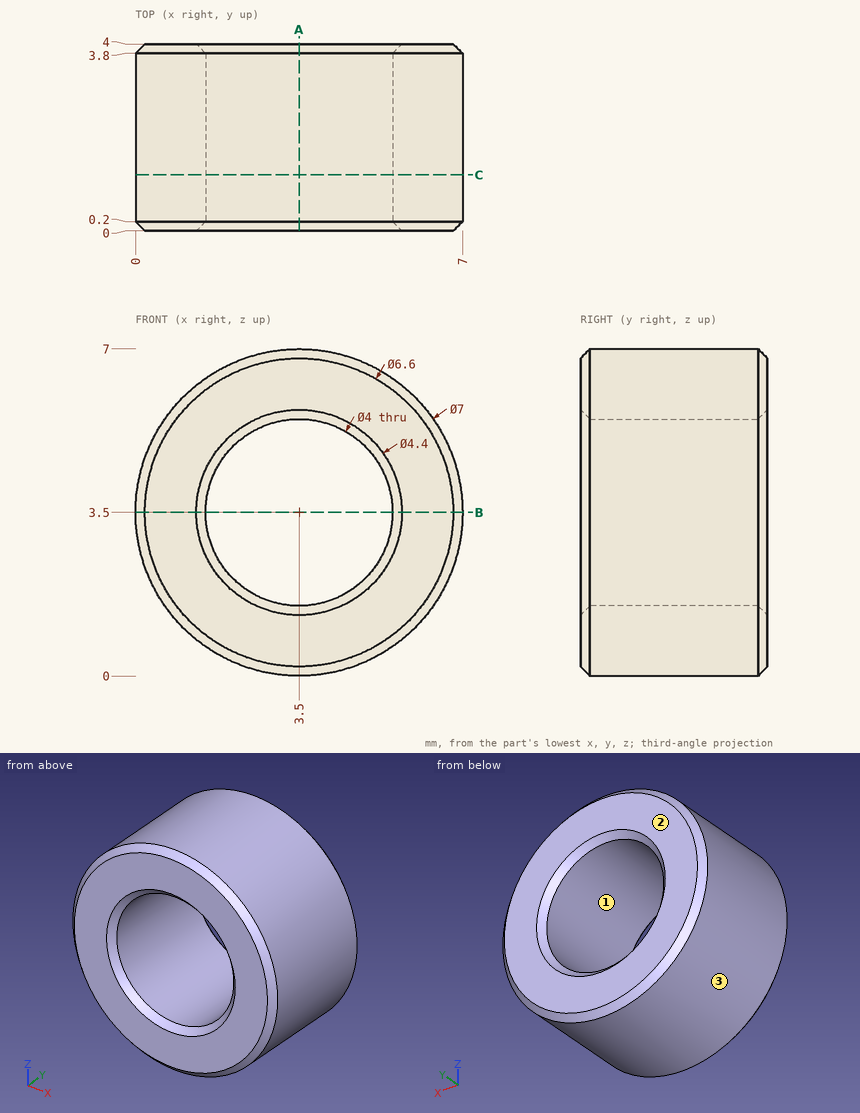
Study the drawing (mm; zero at the part's minimum x, y, z) and answer. Round coordinates to 2 decimals unless told otherwise and drop trailing zeros. Write each loop counter-clockwise with the first axis right and the second up, starting at its lowest first coordinate (ties: lowest second). Pieces come first, ordered by that corner, then holes.
1) A cutting plane is placed at A-A (x = 3.5). Give the vertices of the cut face in (y, z), plus the area to 3 significant figures.
2) The mould has two halves that part along Z. Classify the marked faces 1, 2 and 3: pulls with the +Z half, pulls with the -Z half, needs draft (parallel to the pull), parting line crosses it, or undercut.
3) A cutting plane is placed at C-C (y = 1.2). Give the vertices of the cut face in (x, z), plus the area to 3 significant figures.
4) Straight lines are drawn through the part: line 1 (X direction, y = 2, z = 3.5); line 2 (X direction, y = 1.4, z = 4.75); line 3 (Z direction, x = 3.25, y = 0.65). For each, find the intervals that lie inside material, in ascending order.
5) A cutting plane is placed at B-B (z = 3.5). Give the vertices of the cut face in (x, y), plus the area to 3 significant figures.
6) Given pin 1 Ø3.5 at (x, z) = (3.5, 3.5) entering from +Y, flat-ended and moving along its own axis, determine where the tip first touches the part or whether it passes through.
Completed:
1. outline: (0, 0.2) - (0.2, 0) - (3.8, 0) - (4, 0.2) - (4, 1.3) - (3.8, 1.5) - (0.2, 1.5) - (0, 1.3) - close; (0, 5.7) - (0.2, 5.5) - (3.8, 5.5) - (4, 5.7) - (4, 6.8) - (3.8, 7) - (0.2, 7) - (0, 6.8) - close
1. area: 11.8 mm2
2. face 1: undercut
2. face 2: needs draft
2. face 3: parting line crosses it
3. outline: circle Ø7 at (3.5, 3.5); hole circle Ø4 at (3.5, 3.5)
3. area: 25.9 mm2
4. line 1: x = 0 to 1.5, 5.5 to 7
4. line 2: x = 0.23 to 1.94, 5.06 to 6.77
4. line 3: z = 0.01 to 1.52, 5.48 to 6.99
5. outline: (0, 0.2) - (0.2, 0) - (1.3, 0) - (1.5, 0.2) - (1.5, 3.8) - (1.3, 4) - (0.2, 4) - (0, 3.8) - close; (5.5, 0.2) - (5.7, 0) - (6.8, 0) - (7, 0.2) - (7, 3.8) - (6.8, 4) - (5.7, 4) - (5.5, 3.8) - close
5. area: 11.8 mm2
6. pin 1: passes through
